Source: CAD feature listing. Evaluate the final solid. Frame: model axes, mm. Face numbers are marked on the shaded views. A direction names the side the tool comes from. Coordinates: 2 decimals unless noted, no trailing zeros. Write each loop counter-clockwise with the first axis right and the second up, starting at its lowest first coordinate (ties: lowest second). Pieces come first, ordered by that corner, then holes. Notation, with made-up numbers: M 38.25,65 L 97.25,65 A22 cw 97.25,74 Z; hole C 57,10.25 d8. An arc over 180 degrees is marked long. Write item = value, one per line. Start each with the question number.
1. Access query for the marked faces 1, 2 and 3. Directions: +Z, -Z, +X, -X, +Y, -Y. A direction counts if a zero-diameter tool reaches every point of the face in a straight line with its end or side. Return the directions, or none.
2. Section query A-A (z = -6.35). Output: boundary loops of the cut face in (x, y) (3 decimals).
3. Line query: line 1 along X through (y, z) = (1, -6.35) (3 decimals); line 2 along Y through (x, z) = (5.25, -65); line 3 along Y through (x, z) = (5.5, -7). Output: solid intervals per line, ascending.
4. Pin query (flat end, axial travel): pin 1 Ø3 at (y, z) = (7.5, -31) entering from -X; pin 2 Ø1.6 at (x, z) = (3.18, -49.77) entering from +Y; pin 3 Ø3 at (x, z) = (3.18, -37.07) entering from -Y; pin 4 Ø2.5 at (x, z) = (3.175, -6.35) entering from +Y. Return the tip coordinate at first contact, or that it passes through.
5. Section query B-B (x = 2.75). Output: boundary loops of the cut face in (y, z), then the cut area to 3 significant figures.
6. Section query C-C (z = -22). Output: boundary loops of the cut face in (x, y).
7. Section query D-D (y = 4.25). Output: boundary loops of the cut face in (x, z).
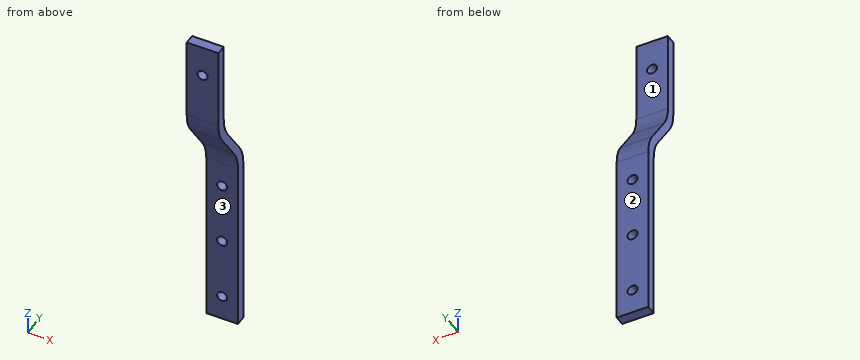
```python
from build123d import *

# Parameters (mm, degrees)
BOSS_EXTRUDE1_DEPTH = 6.35
SKETCH2_R           = 1
CUT_EXTRUDE1_DEPTH  = 2
SKETCH3_R           = 1
CUT_EXTRUDE2_DEPTH  = 2
LPATTERN1_COUNT     = 3
LPATTERN1_PITCH     = 12.7
FILLET1_R           = 7.62


with BuildPart() as part:
    # Sketch1 → Boss-Extrude1 (new body)
    with BuildSketch(Plane(origin=(0, 0, 0), x_dir=(0, 0, -1), z_dir=(1, 0, 0))):
        Polygon((0, 2), (19.05, 2), (29.453230962, 9.284420742), (67.553230962, 9.284420742), (67.553230962, 7.284420742), (29.453230962, 7.284420742), (19.05, 0), (0, 0), align=None)
    extrude(amount=BOSS_EXTRUDE1_DEPTH)

    # Sketch2 → Cut-Extrude1 (cut)
    with BuildSketch(Plane(origin=(0, 2, 0), x_dir=(1, 0, 0), z_dir=(0, 1, 0))):
        with Locations((3.175, 6.35)):
            Circle(SKETCH2_R)
    extrude(amount=-CUT_EXTRUDE1_DEPTH, mode=Mode.SUBTRACT)

    # Sketch3 → Cut-Extrude2 (cut)
    with BuildSketch(Plane(origin=(0, 9.284420742, 0), x_dir=(1, 0, 0), z_dir=(0, 1, 0))):
        with Locations((3.175, 62.473230962)):
            Circle(SKETCH3_R)
    cut_extrude2 = extrude(amount=-CUT_EXTRUDE2_DEPTH, mode=Mode.SUBTRACT)

    # LPattern1: Cut-Extrude2 ×3
    with Locations(*[(0, 0, i * LPATTERN1_PITCH) for i in range(1, LPATTERN1_COUNT)]):
        add(cut_extrude2, mode=Mode.SUBTRACT)

    # Fillet1
    fillet1_edges = [part.edges().sort_by_distance(p)[0] for p in [
        (3.175, 2, -19.05),
        (3.175, 9.284420742, -29.453230962),
        (3.175, 7.284420742, -29.453230962),
        (3.175, 0, -19.05),
    ]]
    fillet(fillet1_edges, radius=FILLET1_R)


solid = part.part
```
Results are:
q1.face_1 = +Z, +X, -X, +Y
q1.face_2 = +Z, -Z, +X, -X, +Y
q1.face_3 = -Z, +X, -X, -Y
q2.outline = M 0,0 L 2.175,0 L 2.175,2 L 0,2 Z; M 4.175,0 L 6.35,0 L 6.35,2 L 4.175,2 Z
q3.line_1 = 0 to 2.175, 4.175 to 6.35
q3.line_2 = 7.28 to 9.28
q3.line_3 = 0 to 2
q4.pin_1 = 0
q4.pin_2 = through
q4.pin_3 = 7.28
q4.pin_4 = 2
q5.outline = M 0,-16.65 A7.62 ccw 1.38,-21.02 L 5.91,-27.49 A7.62 cw 7.28,-31.86 L 7.28,-36.17 L 9.28,-36.17 L 9.28,-31.86 A7.62 ccw 7.91,-27.49 L 3.38,-21.02 A7.62 cw 2,-16.65 L 2,-7.26 L 0,-7.26 Z; M 0,-5.44 L 2,-5.44 L 2,0 L 0,0 Z; M 7.28,-67.55 L 9.28,-67.55 L 9.28,-63.38 L 7.28,-63.38 Z; M 7.28,-61.57 L 9.28,-61.57 L 9.28,-50.68 L 7.28,-50.68 Z; M 7.28,-48.87 L 9.28,-48.87 L 9.28,-37.98 L 7.28,-37.98 Z
q5.area = 121 mm^2
q6.outline = M 0,2.07 L 6.35,2.07 L 6.35,4.07 L 0,4.07 Z
q7.outline = M 0,-25.12 L 6.35,-25.12 L 6.35,-22.26 L 0,-22.26 Z
